Geometry: see drawing. Coordinates: mm, zero at the bounding-box minimum. Give positions to 0.01 mm unless a question says otherwise; leave off trailing zeros. Write each loop counter-clockwise with the first axis right and the second up, starting at its lowest first coordinate (ties: lowest second). Pieces come first, ordered by that corner, then holes. Notation, with made-up numbers: (39.25, 1.5) - (83.25, 1.5) arc R24 cw to (83.25, 39.5) - close; hole circle Ø11 at (81, 37.25). An arc over 180 degrees is marked (long way). Return JSON: item names as keys, results as strings.
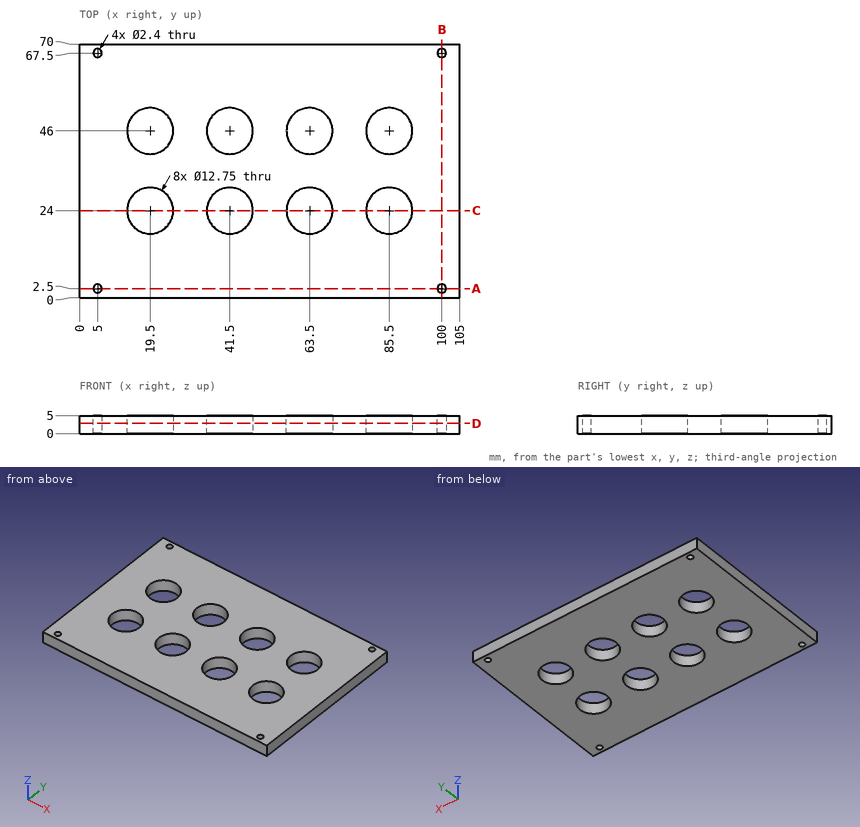
Q1. Material intervals for probe 1 along Y at (x, z) = (63.5, 2.15) (3 decimals); probe 2 along X at (y, z) = (67.5, 2.3); probe 3 along Y at (x, z) = (5, 1.75), sorted ascending. Write a range as [from, to].
Answer key:
{"probe 1": "y = [0, 17.625], [30.375, 39.625], [52.375, 70]", "probe 2": "x = [0, 3.8], [6.2, 98.8], [101.2, 105]", "probe 3": "y = [0, 1.3], [3.7, 66.3], [68.7, 70]"}
Q2. Section query D-D, the plane z = 2.85. Count the separate pieces of the cut face and the enclosed holes in it, plus the area to 3 significant figures.
Answer key:
{"separate pieces": "1", "enclosed holes": "12", "area": "6,310 mm^2"}
Q3. Section query A-A, the plane y = 2.5. Return the cut outline in (x, z).
Answer key:
{"outline": "(0, 0) - (3.8, 0) - (3.8, 5) - (0, 5) - close; (6.2, 0) - (98.8, 0) - (98.8, 5) - (6.2, 5) - close; (101.2, 0) - (105, 0) - (105, 5) - (101.2, 5) - close"}
Q4. Section query C-C, the plane y = 24. Return the cut outline in (x, z) (3 decimals), plus the area to 3 significant figures.
Answer key:
{"outline": "(0, 0) - (13.125, 0) - (13.125, 5) - (0, 5) - close; (25.875, 0) - (35.125, 0) - (35.125, 5) - (25.875, 5) - close; (47.875, 0) - (57.125, 0) - (57.125, 5) - (47.875, 5) - close; (69.875, 0) - (79.125, 0) - (79.125, 5) - (69.875, 5) - close; (91.875, 0) - (105, 0) - (105, 5) - (91.875, 5) - close", "area": "270 mm^2"}
Q5. Section query B-B, the plane x = 100. Return the cut outline in (y, z), plus the area to 3 significant figures.
Answer key:
{"outline": "(0, 0) - (1.3, 0) - (1.3, 5) - (0, 5) - close; (3.7, 0) - (66.3, 0) - (66.3, 5) - (3.7, 5) - close; (68.7, 0) - (70, 0) - (70, 5) - (68.7, 5) - close", "area": "326 mm^2"}
